from build123d import *

# Parameters (mm, degrees)
SKETCH1_R             = 10.05
SKETCH1_R_2           = 1.5
EXTRUSION1_DEPTH      = 18
SKETCH2_R             = 10.05
SKETCH2_R_2           = 1.5
EXTRUSION2_DEPTH      = 13
SKETCH3_R             = 10.05
SKETCH3_R_2           = 1.5
EXTRUSION3_DEPTH      = 9
EXTRUSION4_START      = -4
EXTRUSION4_DEPTH      = 4
SKETCH5_R             = 6.05
SKETCH5_R_2           = 1.5
EXTRUSION5_DEPTH      = 7
SKETCH6_R             = 3.175
SKETCH6_R_2           = 1.5
EXTRUSION6_DEPTH      = 22
EXTRUSION7_DEPTH      = 4.5
SKETCH8_W             = 1.5
SKETCH8_H             = 11.05
EXTRUSION8_DEPTH      = 50.316376633
EXTRUSION8_DEPTH_BACK = 50.316376633
CHAMFER1_SIZE         = 0.4
SKETCH12_W            = 4
SKETCH12_H            = 3
CHAMFER2_SIZE         = 1.6
CHAMFER3_SIZE         = 0.5
CHAMFER4_SIZE         = 0.5
EXTRUSION10_START     = 1
EXTRUSION10_DEPTH     = 1


with BuildPart() as part:
    # Sketch1 → Extrusion1 (new body)
    with BuildSketch(Plane.XY):
        with Locations((0, 1)):
            Circle(SKETCH1_R)
        Circle(SKETCH1_R_2, mode=Mode.SUBTRACT)
    extrude(amount=EXTRUSION1_DEPTH)

    # Sketch2 → Extrusion2 (add)
    with BuildSketch(Plane(origin=(0, 1, 18), x_dir=(1, 0, 0), z_dir=(0, 0, 1))):
        with Locations(Location((0, -2, 0), (0, 0, 174.289477772))):
            Circle(SKETCH2_R)
        with Locations((0, -1)):
            Circle(SKETCH2_R_2, mode=Mode.SUBTRACT)
    extrude(amount=EXTRUSION2_DEPTH)

    # Sketch3 → Extrusion3 (add)
    with BuildSketch(Plane(origin=(0, -1, 31), x_dir=(1, 0, 0), z_dir=(0, 0, 1))):
        with Locations(Location((0, 2, 0), (0, 0, 185.710522228))):
            Circle(SKETCH3_R)
        with Locations((0, 1)):
            Circle(SKETCH3_R_2, mode=Mode.SUBTRACT)
    extrude(amount=EXTRUSION3_DEPTH)

    # Sketch4 → Extrusion4 (cut)
    with BuildSketch(Plane(origin=(0, 1, 31), x_dir=(1, 0, 0), z_dir=(0, 0, 1)).offset(EXTRUSION4_START)):
        with BuildLine():
            ThreePointArc((-10.000124999, -1), (0, -12.05), (10.000124999, -1))
            ThreePointArc((10.000124999, -1), (0, -10.05), (-10.000124999, -1))
        make_face()
    extrude(amount=EXTRUSION4_DEPTH, mode=Mode.SUBTRACT)

    # Sketch5 → Extrusion5 (add)
    with BuildSketch(Plane(origin=(0, 1, 40), x_dir=(1, 0, 0), z_dir=(0, 0, 1))):
        with Locations((0, -1)):
            Circle(SKETCH5_R)
        with Locations((0, -1)):
            Circle(SKETCH5_R_2, mode=Mode.SUBTRACT)
    extrude(amount=EXTRUSION5_DEPTH)

    # Sketch6 → Extrusion6 (cut)
    with BuildSketch(Plane(origin=(0, 1, 0), x_dir=(-1, 0, 0), z_dir=(0, 0, -1))):
        with Locations((0, -1)):
            Circle(SKETCH6_R)
        with Locations((0, -1)):
            Circle(SKETCH6_R_2, mode=Mode.SUBTRACT)
    extrude(amount=-EXTRUSION6_DEPTH, mode=Mode.SUBTRACT)

    # Sketch7 → Extrusion7 (cut)
    with BuildSketch(Plane(origin=(0, 0, 0), x_dir=(-1, 0, 0), z_dir=(0, 1, 0))):
        Polygon((-2.75, 7.41228676), (-2.75, 10.58771324), (0, 12.175426481), (2.75, 10.58771324), (2.75, 7.41228676), (0, 5.824573519), align=None)
    extrude(amount=EXTRUSION7_DEPTH, mode=Mode.SUBTRACT)

    # Sketch8 → Hole2 (revolve, cut)
    with BuildSketch(Plane(origin=(0, 0, 9), x_dir=(0, 0, -1), z_dir=(1, 0, 0))):
        with Locations((0.75, 5.525)):
            Rectangle(SKETCH8_W, SKETCH8_H)
    revolve(axis=Axis((0, 110, 9), (0, -1, 0)), mode=Mode.SUBTRACT)

    # Sketch10 → Extrusion8 (cut, two sides: drawn at the far end of the back side and taken through both)
    with BuildSketch(Plane(origin=(0, 0, 0), x_dir=(-1, 0, 0), z_dir=(0, 1, 0)).offset(-EXTRUSION8_DEPTH_BACK)):
        Polygon((-7.5, 10.707106781), (-8.207106781, 10), (-7.5, 9.292893219), (-6.792893219, 10), align=None)
        Polygon((7.5, 10.707106781), (6.792893219, 10), (7.5, 9.292893219), (8.207106781, 10), align=None)
    extrude(amount=EXTRUSION8_DEPTH + EXTRUSION8_DEPTH_BACK, mode=Mode.SUBTRACT)

    # Chamfer1
    chamfer1_edges = [part.edges().sort_by_distance(p)[0] for p in [
        (10.000124999, 2, 40),
    ]]
    chamfer(chamfer1_edges, length=CHAMFER1_SIZE)

    # Sketch12 → Revolution1 (revolve, cut)
    with BuildSketch(Plane.YZ, mode=Mode.PRIVATE) as revolution1_sk:
        with Locations((-11.05, 1.5)):
            Rectangle(SKETCH12_W, SKETCH12_H)
        Polygon((-9.05, 3), (-13.05, 7), (-13.05, 3), align=None)
    revolve(revolution1_sk.sketch.rotate(Axis((0, 0, -4.4), (0, 0, 1)), 270), axis=Axis((0, 0, -4.4), (0, 0, 1)), mode=Mode.SUBTRACT)

    # Chamfer2
    chamfer2_edges = [part.edges().sort_by_distance(p)[0] for p in [
        (-1.5, 0, 22),
    ]]
    chamfer(chamfer2_edges, length=CHAMFER2_SIZE)

    # Chamfer3
    # the kernel refuses this chamfer: 0.5 mm, written as the material it adds along each edge
    with BuildSketch(Plane(origin=(0, -1, 31), x_dir=(0.9995951137043791, -0.028453622938550055, 0), z_dir=(-0.028453622938550055, -0.9995951137043791, 0))) as chamfer3_piece_1_section:
        Polygon((10.05, -CHAMFER3_SIZE), (10.05 + CHAMFER3_SIZE, 0), (10.05, 0), align=None)
    chamfer3_piece_1 = revolve(axis=Axis((0, -1, 31), (0, 0, 1)), revolution_arc=183.260985134, mode=Mode.PRIVATE)
    chamfer3_piece_1 = chamfer3_piece_1 & Plane(origin=(0, 1, 30.761134514), x_dir=(-0.9950373133554516, -0.09950248755867733, 0), z_dir=(0, 0, -1)) * Cylinder(10.05, 43, mode=Mode.PRIVATE)
    add(chamfer3_piece_1)

    # Chamfer4
    # the kernel refuses this chamfer: 0.5 mm, written as the material it adds along each edge
    with BuildSketch(Plane(origin=(0, 1, 18), x_dir=(-0.9995951137044771, 0.028453622935110102, 0), z_dir=(0.028453622935110102, 0.9995951137044771, 0))) as chamfer4_piece_1_section:
        Polygon((10.05 + CHAMFER4_SIZE, 0), (10.05, -CHAMFER4_SIZE), (10.05, 0), align=None)
    chamfer4_piece_1 = revolve(axis=Axis((0, 1, 18), (0, 0, 1)), revolution_arc=183.260985134, mode=Mode.PRIVATE)
    chamfer4_piece_1 = chamfer4_piece_1 & Plane(origin=(0, -1, 17.760783503), x_dir=(-0.9950373133554516, 0.09950248755867756, 0), z_dir=(0, 0, -1)) * Cylinder(10.05, 43, mode=Mode.PRIVATE)
    add(chamfer4_piece_1)

    # Sketch13 → Extrusion10 (add)
    with BuildSketch(Plane(origin=(0, -1, 31), x_dir=(-1, 0, 0), z_dir=(0, 0, -1)).offset(EXTRUSION10_START)):
        with BuildLine():
            ThreePointArc((9.925818606, 3.575), (0, 12.05), (-9.925818606, 3.575))
            ThreePointArc((-9.925818606, 3.575), (0, 10.55), (9.925818606, 3.575))
        make_face()
    extrude(amount=-EXTRUSION10_DEPTH)


solid = part.part
The listing builds one solid part. Answer for the finished solid, in the listing's coordinates (mm). A direction names the side the tool comes from. Round coordinates to 2 decimals unless told otherwise and drop trailing zeros. Loops run counter-clockwise (first coordinate to the right, second up) from the corner with the lowest first, then second, coordinate; pieces in that order, holes last. Notation, with made-up numbers: M -18,-19 L 20,-19 A17 ccw 20,1 Z; hole C 25.25,79 d4. An arc over 180 degrees is marked long. Write each question's results on one line, items separated by ' | '. Start each with the question number.
1) Find section A-A on y = 1. Count the separate pieces of the cut face and the enclosed holes in it, plus the area to 3 significant figures.
2) Straight lines are drawn through the part: probe 1 along Z at (x, y) = (7.25, 7); probe 2 along Z at (x, y) = (0, 6.25); probe 3 along Y at (x, z) = (0, 39.5). For each, find the intervals that lie inside material, in ascending order.
3) Each of these flat-tipped pins is pushed along its axis until it touches: pin 1 (3 mm diameter, centred on y = 8.5, z = 8, fed in from -X); pin 2 (12 mm diameter, centred on x = 0.5, z = 12.5, fed in from -Y); pin 3 (0.9 mm diameter, centred on y = 2.5, z = 8.5, fed in from -X) (3 decimals); pin 4 (1.5 mm diameter, centred on y = 2.5, z = 9.5, fed in from +X). Where does it stop, or does it pass through?
4) Which of the six approach directions +Z, -Z, +X, -X, +Y, -Y give full straight-line access (tool end or side, diameter ignored) to faces 4 (the flat face through (-0.05, 9.23, 18)), 5 (the cylindrical face through (0.18, 9.55, 30.49)), 6 (the flat face through (-5, 5, 40))?
5) Determine the mould class of faces 1 (the conical face through (-0.21, -9.183, 17.635)), 2 (the flat face through (1, -10, 18)), 3 (the flat face through (1.661, 3.67, 6.784)) for opening direction Y: pulls with the +Y half, pulls with the -Y half, needs draft (parallel to the pull), parting line crosses it, or undercut.
6) Find section B-B on z = 24.5. Write down the section's boundary in (x, y).
Final values:
1) separate pieces: 2 | enclosed holes: 2 | area: 681 mm²
2) probe 1: 4.03 to 9.54, 10.46 to 18, 30 to 40 | probe 2: 0 to 7.5, 10.5 to 40 | probe 3: -9.05 to -1.5, 1.5 to 11.05
3) pin 1: x = -8.06 | pin 2: y = -11.05 | pin 3: x = -9.995 | pin 4: x = 10.02
4) face 4: +Y | face 5: none | face 6: +Z
5) face 1: pulls with the -Y half | face 2: needs draft | face 3: undercut
6) outline: C 0,-1 d20.1; hole C 0,0 d3
